Part model, mm, in its own coordinate system. Face numbers are marked on the shaded views. A direction names the side the tool comes from. Round coordinates to 2 decimals unless told otherwise and drop trailing zeros. Loops run counter-clockwise (first coordinate to the right, second up) from the corner with the lowest first, then second, coordinate; pieces in that order, holes last. Notation, with made-up numbers: (22, -10.75) - (27, -10.75) arc R20 ccw to (27, 7.25) - close; hole circle Ø5 at (58, -25.5). An arc over 180 degrees is marked (long way). Write each question's results on one line, items separated by ' | '. Start each with the question number.
(1) Drill centre lines: L1, parallel to Z at x = -5.25, y = 1.55; L2, parallel to Z at x = 0, y = 3.05; L3, parallel to X at y = 3.5, z = -12. Where is each one in solid material? Low to high.
(2) Cut at D-D, the plane x = 3. List the corners of the cut face in (y, z).
(3) Cut at C-C, the plane z = 4. List the corners of the cut face in (x, y), then the cut area to 3 significant figures.
(4) Mould opens along Z. For the marked faces 1, 2 and 3 say: released by +Z, released by -Z, zero draft, split by the parting line, or undercut.
(5) Tool access for the marked faces 4, 5 and 6: list every direction of +Z, -Z, +X, -X, +Y, -Y with a clear straight run to the whole face (end or side of a thin tool).
(6) Cut at B-B, the plane x = 0.5. List the corners of the cut face in (y, z).
(7) Flat gauge pins, fed straight in: P1, Ø2, axis at x = -7, y = 2.5, coming from the +Z side; P2, Ø0.9, axis at y = 2, z = -1, coming from the -X side; P3, Ø4.5, axis at x = 0, z = 0, coming from the +Y side. Where does each tip first touch, or does it go through?
(8) Cut at A-A, the plane y = 1.85. List the corners of the cut face in (x, z).
from build123d import *

# Parameters (mm, degrees)
SKETCH1_R           = 2
BOSS_EXTRUDE1_DEPTH = 4
CHAMFER1_SIZE       = 6
FILLET1_R           = 3


with BuildPart() as part:
    # Sketch1 → Boss-Extrude1 (new body)
    with BuildSketch(Plane(origin=(0, 0, 0), x_dir=(1, 0, 0), z_dir=(0, 1, 0))):
        with BuildLine():
            ThreePointArc((-5, 0), (0, -5), (5, 0))
            Line((5, 0), (5, 15))
            Line((5, 15), (-9, 15))
            Line((-9, 15), (-9, 11))
            Line((-9, 11), (-5, 11))
            Line((-5, 11), (-5, 7))
            Line((-5, 7), (-9, 7))
            Line((-9, 7), (-9, 3))
            Line((-9, 3), (-5, 3))
            Line((-5, 3), (-5, 0))
        make_face()
        Circle(SKETCH1_R, mode=Mode.SUBTRACT)
    extrude(amount=BOSS_EXTRUDE1_DEPTH)

    # Chamfer1
    chamfer1_edges = [part.edges().sort_by_distance(p)[0] for p in [
        (5, 2, -15),
    ]]
    chamfer(chamfer1_edges, length=CHAMFER1_SIZE)

    # Fillet1
    fillet1_edges = [part.edges().sort_by_distance(p)[0] for p in [
        (-1, 2, -15),
        (5, 2, -9),
    ]]
    fillet(fillet1_edges, radius=FILLET1_R)


solid = part.part
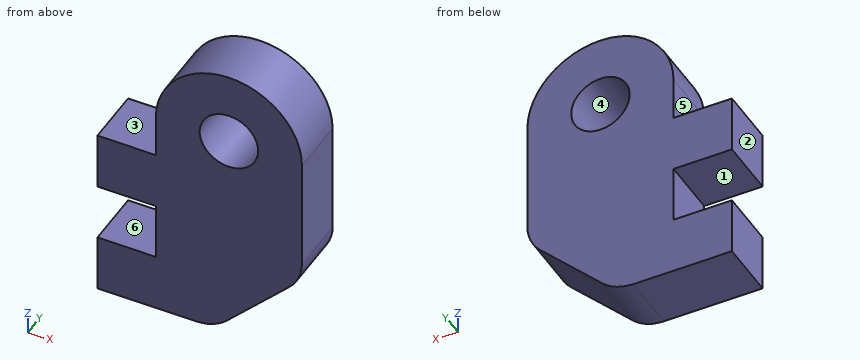
A:
1) L1: -15 to -11, -7 to -3 | L2: -14 to -2, 2 to 5 | L3: -9 to 2
2) outline: (0, -11) - (4, -11) - (4, 4) - (0, 4) - close
3) outline: (-3, 0) - (3, 0) - (3, 4) - (-3, 4) - close | area: 24.0 mm2
4) face 1: undercut | face 2: zero draft | face 3: released by +Z
5) face 4: +Y, -Y | face 5: +Z, -X, +Y, -Y | face 6: -X, +Y, -Y
6) outline: (0, -13.5) - (4, -13.5) - (4, -1.94) - (0, -1.94) - close; (0, 1.94) - (4, 1.94) - (4, 4.97) - (0, 4.97) - close
7) P1: z = -3 | P2: x = -5 | P3: y = 4
8) outline: (-9, -15) - (-2.24, -15) arc R3 ccw to (-0.12, -14.12) - (4.12, -9.88) arc R3 ccw to (5, -7.76) - (5, 0) arc R5 ccw to (-5, 0) - (-5, -3) - (-9, -3) - (-9, -7) - (-5, -7) - (-5, -11) - (-9, -11) - close; hole circle Ø4 at (0, 0)
